```python
from build123d import *

# Parameters (mm, degrees)
PAD_DEPTH    = 25
SKETCH001_R  = 2
POCKET_DEPTH = 6


with BuildPart() as part:
    # Sketch → Pad (new body, symmetric)
    with BuildSketch(Plane.XY):
        Polygon((0, -4.618802), (4, -2.309401), (4, 2.309401), (0, 4.618802), (-4, 2.309401), (-4, -2.309401), align=None)
    extrude(amount=PAD_DEPTH, both=True)

    # Sketch001 (on Face8 of Pad) → Pocket (cut)
    with BuildSketch(Plane.XY.offset(25)):
        Circle(SKETCH001_R)
    pocket = extrude(amount=-POCKET_DEPTH, mode=Mode.SUBTRACT)

    # Mirrored: Pocket across XY
    add(pocket.mirror(Plane.XY), mode=Mode.SUBTRACT)


solid = part.part
```
Work out the finished part from the listing and answer in its coordinate system (mm). A direction names the side the tool comes from. Round coordinates to 2 decimals unless told otherwise and drop trailing zeros. Loops run counter-clockwise (first coordinate to the right, second up) from the corner with the lowest first, then second, coordinate; pieces in that order, holes last. Notation, with made-up numbers: (-37, 26) -> (-12, 26) arc R16 cw to (-12, 51) -> close; hole circle Ø10 at (-25, -24). An arc over 180 degrees is marked (long way). Write each question's results on one line, items separated by ' | '. Start each with the question number.
1. Find the intervals of material crossed by probe 1 along Y at (x, z) = (0, 23.4); probe 2 along Z at (x, y) = (0.5, 1.5); probe 3 along Y at (x, z) = (0.5, 21.5), in increasing order. Write a range as from..to.
2. Section A-A (z = 20) is taken. Determine the outline of the cut face in (x, y).
3. A tool of negligible diameter and unlimited length cuts with its end or side. For faces 5 (the face through (0, -2, -22)), 6 (the face through (1.97, -3.48, 0.35)), from which of +Z, -Z, +X, -X, +Y, -Y can it reach the whole face along a straight path? Write none if from no direction.
4. For a pull along Y with two mould halves and no side action, classify faces 1 (the face through (2.028, 3.448, 0.35)), 2 (the face through (-4, 0, 0)), 3 (the face through (0, 0, 19)), 4 (the face through (0, -2, 22)) as +Y half, -Y half, draft (parallel to the pull), parting line (faces both ways), or undercut.
5. Section C-C (z = 12) is taken. Determine the outline of the cut face in (x, y).
6. Section B-B (y = 0) is taken. Determine the outline of the cut face in (x, z).
7. Section D-D (x = 1.5) is taken. Determine the outline of the cut face in (y, z), plus the area to 3 significant figures.
8. Given pin 1 Ø1.5 at (x, z) = (-1, 2.5) entering from -Y; pin 2 Ø2.5 at (x, y) = (0, 0) entering from -Z, each flat-ended and moving along its own axis, determine where each tip first touches the part or whether it passes through.
Evaluation:
1) probe 1: y = -4.62..-2, 2..4.62 | probe 2: z = -19..19 | probe 3: y = -4.33..-1.94, 1.94..4.33
2) outline: (-4, -2.31) -> (0, -4.62) -> (4, -2.31) -> (4, 2.31) -> (0, 4.62) -> (-4, 2.31) -> close; hole circle Ø4 at (0, 0)
3) face 5: -Z | face 6: +Z, -Z, +X, -Y
4) face 1: +Y half | face 2: draft | face 3: undercut | face 4: undercut
5) outline: (-4, -2.31) -> (0, -4.62) -> (4, -2.31) -> (4, 2.31) -> (0, 4.62) -> (-4, 2.31) -> close
6) outline: (-4, -25) -> (-2, -25) -> (-2, -19) -> (2, -19) -> (2, -25) -> (4, -25) -> (4, 25) -> (2, 25) -> (2, 19) -> (-2, 19) -> (-2, 25) -> (-4, 25) -> close
7) outline: (-3.75, -25) -> (-1.32, -25) -> (-1.32, -19) -> (1.32, -19) -> (1.32, -25) -> (3.75, -25) -> (3.75, 25) -> (1.32, 25) -> (1.32, 19) -> (-1.32, 19) -> (-1.32, 25) -> (-3.75, 25) -> close | area: 344 mm2
8) pin 1: stops at y = -4.47 | pin 2: stops at z = -19
